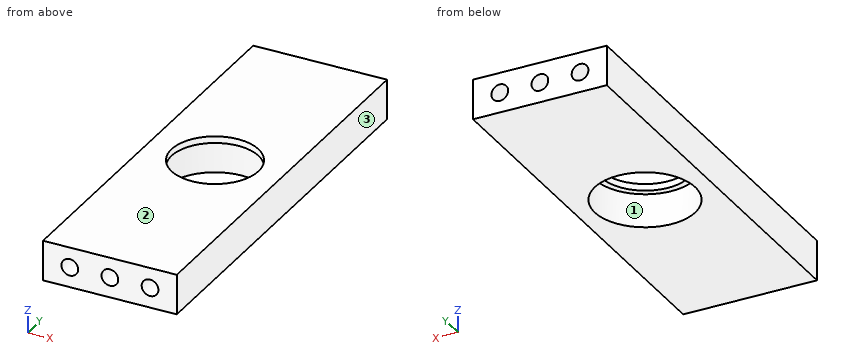
from build123d import *

# Parameters (mm, degrees)
SKETCH_1_R             = 7.5
EXTRUDE_1_DEPTH        = 6
SKETCH_2_R             = 7.5
SKETCH_2_R_2           = 6.5
EXTRUDE_3_DEPTH        = 1
HOLE_WIZARD_M3_1_D     = 2.5
HOLE_WIZARD_M3_1_DEPTH = 10
HOLE_WIZARD_M3_1_TIP   = 0.751075774
HOLE_WIZARD_M3_2_D     = 2.5
HOLE_WIZARD_M3_2_DEPTH = 10
HOLE_WIZARD_M3_2_TIP   = 0.751075774


with BuildPart() as part:
    # 스케치1 → 보스-돌출1 (new body)
    with BuildSketch(Plane.XY):
        Polygon((-7.784090909, 20.710227273), (-7.784090909, -9.289772727), (12.215909091, -9.289772727), (12.215909091, 20.710227273), (12.215909091, 50.710227273), (-7.784090909, 50.710227273), align=None)
        with Locations((2.215909091, 20.710227273)):
            Circle(SKETCH_1_R, mode=Mode.SUBTRACT)
    extrude(amount=EXTRUDE_1_DEPTH)

    # 스케치2 → 보스-돌출3 (add)
    with BuildSketch(Plane.XY.offset(6)):
        with Locations((2.215909091, 20.710227273)):
            Circle(SKETCH_2_R)
        with Locations((2.215909091, 20.710227273)):
            Circle(SKETCH_2_R_2, mode=Mode.SUBTRACT)
    extrude(amount=-EXTRUDE_3_DEPTH)

    # M3 나사 구멍1
    with Locations(Plane(origin=(0, -9.289772727, 0), x_dir=(-1, 0, 0), z_dir=(0, -1, 0))):
        with Locations((3.784090909, -3), (-2.215909091, -3), (-8.215909091, -3)):
            Hole(HOLE_WIZARD_M3_1_D / 2, depth=HOLE_WIZARD_M3_1_DEPTH)
            with Locations((0, 0, -(HOLE_WIZARD_M3_1_DEPTH + HOLE_WIZARD_M3_1_TIP / 2))):  # 118° drill point
                Cone(0, HOLE_WIZARD_M3_1_D / 2, HOLE_WIZARD_M3_1_TIP, mode=Mode.SUBTRACT)

    # M3 나사 구멍2
    with Locations(Plane(origin=(0, 50.710227273, 0), x_dir=(1, 0, 0), z_dir=(0, 1, 0))):
        with Locations((-3.784090909, -3), (2.215909091, -3), (8.215909091, -3)):
            Hole(HOLE_WIZARD_M3_2_D / 2, depth=HOLE_WIZARD_M3_2_DEPTH)
            with Locations((0, 0, -(HOLE_WIZARD_M3_2_DEPTH + HOLE_WIZARD_M3_2_TIP / 2))):  # 118° drill point
                Cone(0, HOLE_WIZARD_M3_2_D / 2, HOLE_WIZARD_M3_2_TIP, mode=Mode.SUBTRACT)


solid = part.part
Design review of the part built by this model. Coordinates are the model's own, in mm. Face numbers are marked on the shaded views. Round coordinates to 2 decimals unless told otherwise and drop trailing zeros. Write each loop counter-clockwise with the first axis right and the second up, starting at its lowest first coordinate (ties: lowest second). Pieces come first, ordered by that corner, then holes. Notation, with made-up numbers: (-38.75, 39.25) - (-2.75, 39.25) arc R13 cw to (-2.75, 64.25) - close; hole circle Ø8 at (50.25, -2.75). An arc over 180 degrees is marked (long way). Return JSON: item names as keys, results as strings. Group by question number.
Item 1: We need section A-A on x = -0.75. Write out the cut boundary in (y, z), and give its area (3 significant figures).
Item 2: We need section C-C on y = 24. Write out the cut boundary in (x, z), and give its area (3 significant figures).
Item 3: We need section B-B on y = 45.5. Write out the cut boundary in (x, z).
Item 4: For probe 1 along Z at (x, y) = (-3.5, 25); probe 2 along Z at (x, y) = (2.5, 46); probe 3 along Y at (x, z) = (6.75, 2.4), list the stretches that pass through material, from the lowest coordinate up. Write a range as [from, to].
Item 5: Insertion check: P1, Ø5, axis at x = 6, y = -3, coming from the -Z side; P2, Ø4.5, axis at x = -0.5, y = 21, coming from the -Z side; P3, Ø2, axis at x = -3.78, z = 3, coming from the +Y side; P4, Ø2, axis at x = 8.22, z = 3, coming from the -Y side. Each pin has a flat end and moves straight along its axis. Give the tip position at first contact, or say it passes through.
Item 6: The part is to be moulded in two halves that separate along X. For the marked faces 1, 2 and 3, say which applies: pulls with the +X half, pulls with the -X half, needs draft (parallel to the pull), parting line crosses it, or undercut.
Model answer:
{
 "1": {"outline": "(-9.29, 0) - (13.82, 0) - (13.82, 5) - (14.93, 5) - (14.93, 6) - (-9.29, 6) - close; (26.49, 5) - (27.6, 5) - (27.6, 0) - (50.71, 0) - (50.71, 6) - (26.49, 6) - close", "area": "280 mm²"},
 "2": {"outline": "(-7.78, 0) - (-4.52, 0) - (-4.52, 5) - (-3.39, 5) - (-3.39, 6) - (-7.78, 6) - close; (7.82, 5) - (8.96, 5) - (8.96, 0) - (12.22, 0) - (12.22, 6) - (7.82, 6) - close", "area": "41.4 mm²"},
 "3": {"outline": "(-7.78, 0) - (12.22, 0) - (12.22, 6) - (-7.78, 6) - close; hole circle Ø2.5 at (-3.78, 3); hole circle Ø2.5 at (2.22, 3); hole circle Ø2.5 at (8.22, 3)"},
 "4": {"probe 1": "z = [5, 6]", "probe 2": "z = [0, 1.78], [4.22, 6]", "probe 3": "y = [-9.29, 14.74], [26.68, 50.71]"},
 "5": {"P1": "stops at z = 0", "P2": "passes through", "P3": "stops at y = 40.56", "P4": "stops at y = 0.86"},
 "6": {"face 1": "undercut", "face 2": "needs draft", "face 3": "pulls with the +X half"}
}
